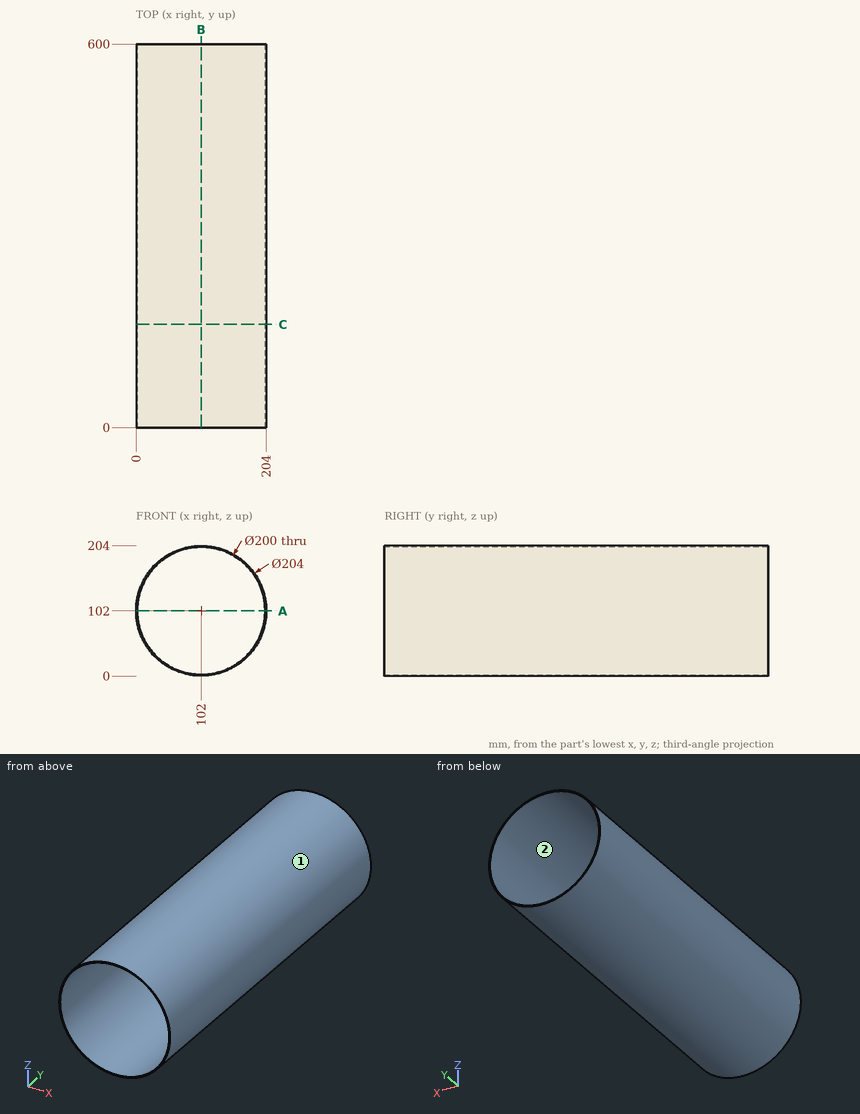
Input: dimensioned drawing with shaded views. Units: mm. Origin: part minimum x, y, z. Round coordinates to 2 decimals unless told otherwise and drop trailing zeros. Order: outer loops, then holes, each group sorted by start corner. A loop starts at its lowest first (then second) coordinate and runs counter-clockwise, first axis right, second up. Notation, with made-up numbers: (42.5, 74) - (71.5, 74) arc R8 cw to (71.5, 80) - close; hole circle Ø7 at (62.5, 36.5). An arc over 180 degrees is marked (long way). Use CSV: the item, a comma, the result in double quotes. Start each with the question number.
Q1. First-contact query: pin 1 (1.5 mm diameter, centred on x = 172, y = 203.5, fed in from +Z); pin 2 (4 mm diameter, centred on x = 38.5, y = 474, fed in from +Z); pin 3 (12 mm diameter, centred on y = 191, z = 137, fed in from -X). Flat tips, straight axial feed; report the tip coordinate or a pass-through.
Q2. Mould query, pull axis X, two halves, no side actions, for the marked faces 1 and 2. Classes: +X half, -X half, draft (parallel to the pull), parting line (faces both ways), or undercut.
Q3. Section query B-B (x = 102). Return loops of the section in (y, z).
Q4. Material intervals for line 1 along Z through (x, y) = (104.5, 132); line 2 along Z through (x, y) = (162.5, 277.5); line 3 along X through (y, z) = (515.5, 24.5), sorted ascending. Write a range as from..to.
Q5. Section query A-A (z = 102). Return loops of the section in (x, y), and give its area (3 significant figures).
Q6. Section query C-C (y = 161.5). Return loops of the section in (x, z), and give its area (3 significant figures).
Result set:
1,pin 1,"stops at z = 176.89"
1,pin 2,"stops at z = 183.37"
1,pin 3,"stops at x = 4.21"
2,face 1,"parting line"
2,face 2,"undercut"
3,outline,"(0, 0) - (600, 0) - (600, 2) - (0, 2) - close; (0, 202) - (600, 202) - (600, 204) - (0, 204) - close"
4,line 1,"z = 0.03..2.03, 201.97..203.97"
4,line 2,"z = 19.88..22.38, 181.62..184.12"
4,line 3,"x = 35.68..38.8, 165.2..168.32"
5,outline,"(0, 0) - (2, 0) - (2, 600) - (0, 600) - close; (202, 0) - (204, 0) - (204, 600) - (202, 600) - close"
5,area,"2,400 mm2"
6,outline,"circle Ø204 at (102, 102); hole circle Ø200 at (102, 102)"
6,area,"1,270 mm2"
